Read the model definition and answer for the solid it produces. Units are mm, in the model's axes. Round coordinates to 2 decimals unless told otherwise and drop trailing zeros. Write each loop counter-clockwise with the first axis right and the second up, starting at its lowest first coordinate (ties: lowest second). Pieces come first, ordered by that corner, then holes. Notation, with made-up numbers: (48, 17.5) - (86, 17.5) arc R28 ccw to (86, 40.5) - close; hole circle Ø11 at (7, 75.25). An arc over 180 degrees is marked (long way). Use one line per item in the form item = value. Start each with the question number.
1) The part is cut by section C-C, the plane x = -1.65. Give the vertices of the cut face in (y, z), plus the area to 3 significant figures.
2) Consider line 1 along Z through (x, y) = (-0.8, -5.5); line 2 along Z through (x, y) = (-1.25, 25); line 3 along Y through (x, z) = (-2.65, -31). Determine where each line is inside the solid, lowest interval first. Write a range as from..to.
3) This flat-tipped pin is pushed along its axis until it touches: pin 1 (2.5 mm diameter, centred on y = -5.5, z = -25, fed in from -X). Where does it stop, or does it pass through?
4) The part is cut by section A-A, the plane z = -31. Give the vertices of the cut face in (x, y), plus the area to 3 significant figures.
5) The part is cut by section B-B, the plane y = -5.5. Give the vertices of the cut face in (x, z).
from build123d import *

# Parameters (mm, degrees)
SKETCH_1_W          = 4
SKETCH_1_H          = 80
EXTRUDE_3_DEPTH     = 120
SKETCH_3_R          = 2
CUT_EXTRUDE_1_DEPTH = 131.061523903
EXTRUDE_4_DEPTH     = 80


with BuildPart() as part:
    # 草图1 → 拉伸3 (new body)
    with BuildSketch(Plane.XY):
        with Locations((-2, 10)):
            Rectangle(SKETCH_1_W, SKETCH_1_H)
    extrude(amount=-EXTRUDE_3_DEPTH)

    # 草图3 → 切除-拉伸1 (cut, through all)
    with BuildSketch(Plane.ZY.offset(4)):
        with Locations(Location((-89, 25, 0), (0, 0, 270))):
            Circle(SKETCH_3_R)
        with Locations(Location((-95, -5.5, 0), (0, 0, 270))):
            Circle(SKETCH_3_R)
        with Locations(Location((-25, -5.5, 0), (0, 0, 90))):
            Circle(SKETCH_3_R)
        with Locations(Location((-31, 25, 0), (0, 0, 90))):
            Circle(SKETCH_3_R)
    extrude(amount=-CUT_EXTRUDE_1_DEPTH, mode=Mode.SUBTRACT)

    # 草图4 → 拉伸4 (add)
    with BuildSketch(Plane(origin=(0, 50, 0), x_dir=(-1, 0, 0), z_dir=(0, 1, 0))):
        Polygon((4, 0), (0, 1.656854249), (0, 0), align=None)
        Polygon((4, -120), (0, -120), (0, -121.656854249), align=None)
    extrude(amount=-EXTRUDE_4_DEPTH)


solid = part.part
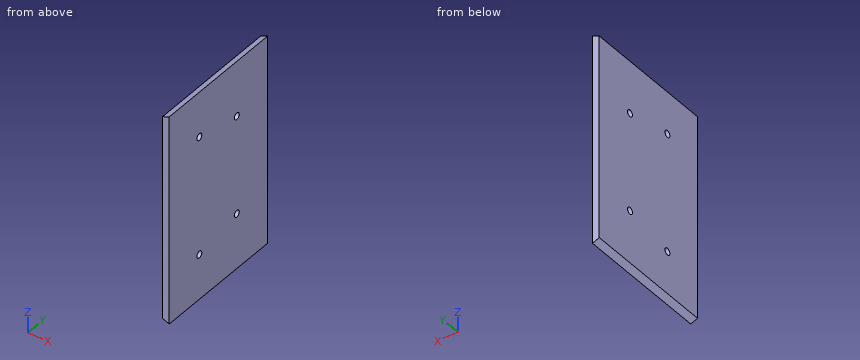
Geometry results:
q1.outline = (-30, -120.97) - (50, -120.97) - (50, 0.97) - (-30, 0.97) - close; hole circle Ø4 at (-5.5, -95); hole circle Ø4 at (-5.5, -25); hole circle Ø4 at (25, -89); hole circle Ø4 at (25, -31)
q1.area = 9,710 mm2
q2.line_1 = -121.33..-97, -93..-27, -23..1.33
q2.line_2 = -121.14..-91, -87..-33, -29..1.14
q2.line_3 = -30..23, 27..50
q3.pin_1 = through
q4.outline = (-4, -30) - (0, -30) - (0, 23) - (-4, 23) - close; (-4, 27) - (0, 27) - (0, 50) - (-4, 50) - close
q4.area = 304 mm2
q5.outline = (-4, -120) - (0, -121.66) - (0, -97) - (-4, -97) - close; (-4, -93) - (0, -93) - (0, -27) - (-4, -27) - close; (-4, -23) - (0, -23) - (0, 1.66) - (-4, 0) - close
